Read the model definition and answer for the solid it produces. Units are mm, in the model's axes. Coordinates: 2 decimals unless noted, no trailing zeros. Write each loop counter-clockwise with the first axis right and the second up, starting at its lowest first coordinate (ties: lowest second). Pieces come first, ordered by that corner, then holes. Notation, with made-up numbers: M -6.75,31.5 L 41.25,31.5 A15 cw 41.25,53.5 Z; hole C 71.25,62.5 d4. An arc over 180 degrees is marked long. Use a Markdown table: item, result. Add a question column.
from build123d import *

# Parameters (mm, degrees)
F0_W     = 34
F0_H     = 70
F1_DEPTH = 13
F2_R     = 6.49999
F3_R     = 6.49999


# Not quite as in the source:
# - a fillet or chamfer is up to 0.001 mm smaller than in the source, because OpenCascade refuses the exact size


with BuildPart() as f1:
    # F0 (on Top) → F1 (new body)
    with BuildSketch(Plane.XY):
        with Locations((17, 35)):
            Rectangle(F0_W, F0_H)
    extrude(amount=F1_DEPTH)

    # F2 (radius 6.5 in the source; OpenCascade refuses exactly that, so slightly less here)
    f2_edges = [f1.edges().sort_by_distance(p)[0] for p in [
        (17, 0, 13),
        (17, 0, 0),
    ]]
    fillet(f2_edges, radius=F2_R)

    # F3 (radius 6.5 in the source; OpenCascade refuses exactly that, so slightly less here)
    f3_edges = [f1.edges().sort_by_distance(p)[0] for p in [
        (17, 70, 13),
        (17, 70, 0),
    ]]
    fillet(f3_edges, radius=F3_R)


solid = f1.part
Item 1: Find section C-C on z = 11.5. Give the vertices of the cut face in (x, y).
Item 2: Each of these flat-tipped pins is pushed along its axis until it touches: pin 1 (1.5 mm diameter, centred on x = 7.5, z = 9.5, fed in from -Y); pin 2 (4 mm diameter, centred on x = 14, z = 3.5, fed in from -Y). Where does it stop, or does it pass through?
Item 3: Find section B-B on z = 1.75. Give the vertices of the cut face in (x, y).
Item 4: Consider probe 1 along Y at (x, z) = (12.5, 3.5); probe 2 along Y at (x, z) = (17, 9); probe 3 along Z at (x, y) = (21, 6). Determine where each line is inside the solid, lowest interval first.
Geometry says:
| question | item | result |
|---|---|---|
| 1 | outline | M 0,2.35 L 34,2.35 L 34,67.65 L 0,67.65 Z |
| 2 | pin 1 | stops at y = 0.4 |
| 2 | pin 2 | stops at y = 0.08 |
| 3 | outline | M 0,2.06 L 34,2.06 L 34,67.94 L 0,67.94 Z |
| 4 | probe 1 | y = 0.73 to 69.27 |
| 4 | probe 2 | y = 0.5 to 69.5 |
| 4 | probe 3 | z = 0.02 to 12.98 |
